Autodesk Inventor part; units mm, degrees
ref_plane "YZ Plane" through (0, 0, 0) normal (1, 0, 0) x (0, 1, 0)
ref_plane "XZ Plane" through (0, 0, 0) normal (0, 1, 0) x (-1, 0, 0)
ref_plane "XY Plane" through (0, 0, 0) normal (0, 0, 1) x (1, 0, 0)
sketch "Sketch1" plane through (0, 0, 0) normal (0, 0, 1) x (1, 0, 0)
  line L0 (0, 0) -> (40, 0)
  line L1 (40, 0) -> (40, 40)
  line L2 (40, 40) -> (0, 40)
  line L3 (0, 40) -> (0, 0)
extrude "Extrusion1" add sketch "Sketch1" along normal blind 20
sketch "Sketch2" plane through (0, 0, 0) normal (0, 0, 1) x (1, 0, 0)
  point P0 (20, 20)
hole "Hole1" at (20, 20, 0) direction (0, 0, 1) diameter 6 end through all counterbore diameter 14 counterbore depth 5
properties part number "25_hole_counterbore"
Can you work these out from the model? Positions are in its coordinate system, mm. A direction names the side the tool comes from. Coordinates: 2 decimals unless noted, no trailing zeros. Write each loop counter-clockwise with the first axis right and the second up, starting at its lowest first coordinate (ties: lowest second). Pieces come first, ordered by that corner, then holes. Notation, with made-up numbers: M -39,62.25 L -27,62.25 A16 cw -27,92.25 Z; hole C 17.5,47.25 d3. An arc over 180 degrees is marked long. Write item = value, one per line. Start each with the question number.
Q1. If we section it at C-C, the plane z = 3.5: Write out the boundary of the cut face in (x, y).
Q2. I'm going to push a flat-ended pin straight in: pin 1 (4 mm diameter, centred on x = 20.5, y = 18, fed in from -Z). Where does the tip first touch, or does it pass through?
Q3. Thinking about a two-plate mould opening in Y: for faces 1 (the face through (20, 0, 10)), 2 (the face through (20, 13, 3)), 3 (the face through (29, 20, 0)), which applies, released by +Y, released by -Y, zero draft, split by the parting line, or undercut?
Q4. If I drill on L1, parallel to X at y = 20, z = 10.25; L2, parallel to X at y = 20, z = 3.5, over which ranges is the centre line in solid material (lowest first)? Write a range as [from, to].
Q5. If we section it at D-D, the plane x = 25: Write out the boundary of the cut face in (y, z), then the cut area to 3 significant figures.
Q6. If we section it at A-A, the plane x = 20: Write out the boundary of the cut face in (y, z).
Q7. On a 3-axis mill with a long thin cutter (end or side, diameter ignored), from which of +Z, -Z, +X, -X, +Y, -Y can I reach the whole of each face in a straight line? I mean faces 4 (the face through (21.8, 17.6, 12.6)), 5 (the face through (21, 23, 5)). Say none if no direction works.
Check sheet entries:
q1.outline = M 0,0 L 40,0 L 40,40 L 0,40 Z; hole C 20,20 d14
q2.pin_1 = 5
q3.face_1 = released by -Y
q3.face_2 = undercut
q3.face_3 = zero draft
q4.L1 = [0, 17], [23, 40]
q4.L2 = [0, 13], [27, 40]
q5.outline = M 0,0 L 15.1,0 L 15.1,5 L 24.9,5 L 24.9,0 L 40,0 L 40,20 L 0,20 Z
q5.area = 751 mm²
q6.outline = M 0,0 L 13,0 L 13,5 L 17,5 L 17,20 L 0,20 Z; M 23,5 L 27,5 L 27,0 L 40,0 L 40,20 L 23,20 Z
q7.face_4 = +Z, -Z
q7.face_5 = -Z
